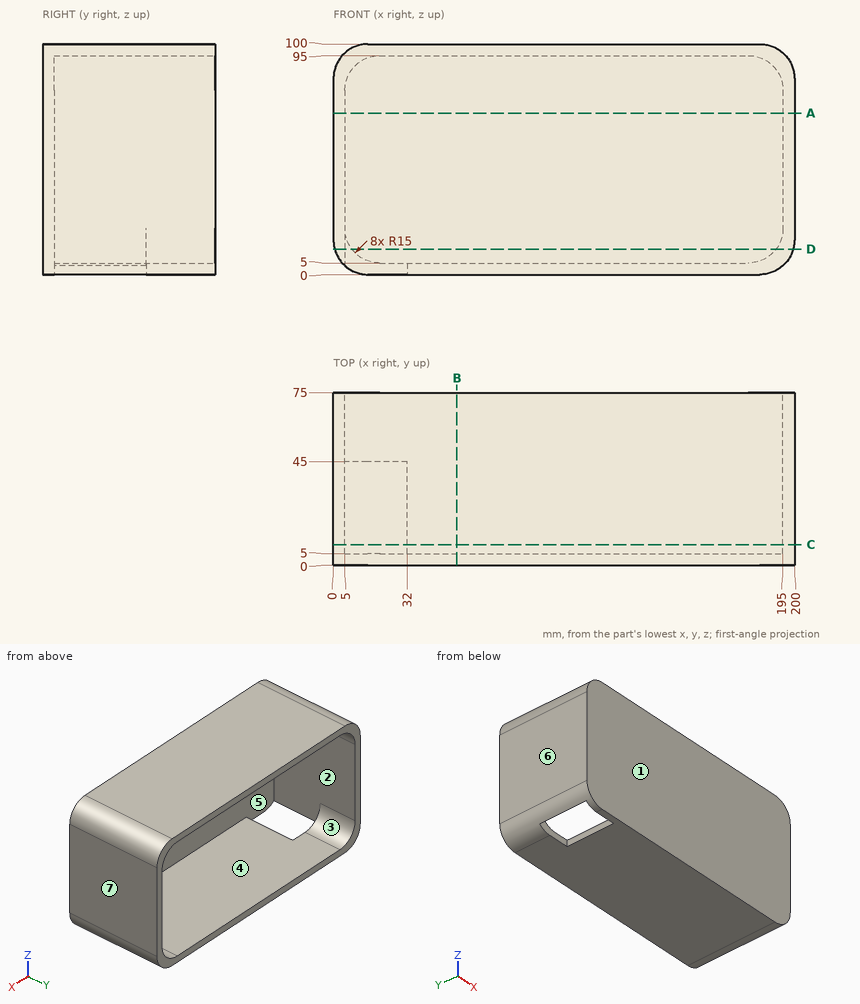
Geometry: see drawing. Coordinates: mm, zero at the bounding-box minimum. A direction names the side the tool comes from. Give positions to 0.01 mm unless a question says otherwise; leave off trailing zeros. Loops run counter-clockwise (first coordinate to the right, second up) from the corner with the lowest first, then second, coordinate; pieces in that order, holes last. Notation, with made-up numbers: (12, 85.5) - (52, 85.5) arc R12 ccw to (52, 108.5) - close; hole circle Ø2 at (-5, 12). An arc over 180 degrees is marked (long way). Answer as CSV lines item,"result". Start each with the question number.
1. Pin query (flat end, axial travel): P1, Ø6, axis at x = 160, z = 43.5, coming from the +Y side; P2, Ø4, axis at y = 15, z = 3, coming from the -X side. Return the tip coordinate at first contact, or that it passes through.
2. Section C-C, the plane y = 9. Return loops of the section in (x, z), plus the area to 3 significant figures.
3. Reachability of the marked faces 1, 2 and 3 from +Z, -Z, +X, -X, +Y, -Y: full face, straight path, thin tool, end or side. Return the list, or none.
4. Ray query, L1, parallel to Z at x = 90, y = 6.5; L2, parallel to X at y = 33.5, z = 31.5; L3, parallel to Y at x = 162.5, z = 6.5. Return the intervals inside material, ascending.
5. Section A-A, the plane z = 70. Return loops of the section in (x, y).
6. Section B-B, the plane x = 53.5. Return loops of the section in (y, z).
7. Section D-D, the plane z = 11. Return loops of the section in (x, y), plus the area to 3 significant figures.
8. Draft query along X for the marked faces 4, 5, 6 and 7. Return one class per face: released by +X, released by -X, zero draft, split by the parting line, or undercut.
Answers:
1,P1,"stops at y = 5"
1,P2,"stops at x = 3.82"
2,outline,"(0, 15) arc R15 ccw to (5, 3.82) - (5, 80) arc R15 cw to (20, 95) - (180, 95) arc R15 cw to (195, 80) - (195, 20) arc R15 cw to (180, 5) - (32, 5) - (32, 0) - (185, 0) arc R15 ccw to (200, 15) - (200, 85) arc R15 ccw to (185, 100) - (15, 100) arc R15 ccw to (0, 85) - close"
2,area,"2,730 mm2"
3,face 1,"+Z, -Z, +X, -X, -Y"
3,face 2,"none"
3,face 3,"+Y"
4,L1,"z = 0 to 5, 95 to 100"
4,L2,"x = 0 to 5, 195 to 200"
4,L3,"y = 0 to 5"
5,outline,"(0, 0) - (200, 0) - (200, 75) - (195, 75) - (195, 5) - (5, 5) - (5, 75) - (0, 75) - close"
6,outline,"(0, 0) - (75, 0) - (75, 5) - (5, 5) - (5, 95) - (75, 95) - (75, 100) - (0, 100) - close"
7,outline,"(0.54, 0) - (199.46, 0) - (199.46, 75) - (192, 75) - (192, 5) - (5, 5) - (5, 45) - (8, 45) - (8, 75) - (0.54, 75) - close"
7,area,"1,920 mm2"
8,face 4,"undercut"
8,face 5,"undercut"
8,face 6,"released by -X"
8,face 7,"released by +X"
